Model file for the job. Use its own axes, mm. Face numbers are marked on the shaded views. Round coordinates to 2 decimals unless told otherwise and drop trailing zeros. Write each loop counter-clockwise with the first axis right and the second up, starting at its lowest first coordinate (ties: lowest second). Pieces come first, ordered by that corner, then holes. Notation, with made-up numbers: (52.25, -34.5) - (63.25, -34.5) arc R24 cw to (63.25, -7.5) - close; hole circle Ø3 at (18.25, 73). An arc over 180 degrees is marked (long way). One line per item, written item: value.
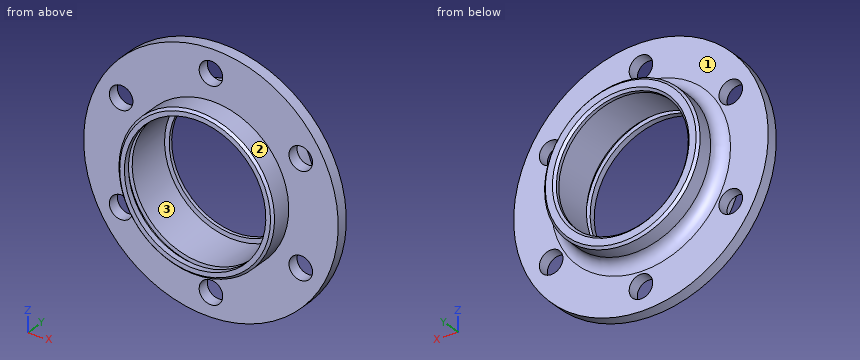
from build123d import *

# Parameters (mm, degrees)
SKETCH1_R           = 27
SKETCH1_R_2         = 2.5
SKETCH1_R_3         = 16.5
BOSS_EXTRUDE1_DEPTH = 2.5
FILLET1_R           = 2.5


with BuildPart() as part:
    # Sketch1 → Boss-Extrude1 (new body)
    with BuildSketch(Plane(origin=(0, 0, 0), x_dir=(1, 0, 0), z_dir=(0, 1, 0))):
        with Locations(Location((0, 0, 0), (0, 0, 270))):
            Circle(SKETCH1_R)
        with Locations(Location((0, 22, 0), (0, 0, 270))):
            Circle(SKETCH1_R_2, mode=Mode.SUBTRACT)
        with Locations(Location((19.052558883, 11, 0), (0, 0, 270))):
            Circle(SKETCH1_R_2, mode=Mode.SUBTRACT)
        with Locations(Location((19.052558883, -11, 0), (0, 0, 270))):
            Circle(SKETCH1_R_2, mode=Mode.SUBTRACT)
        with Locations(Location((0, -22, 0), (0, 0, 270))):
            Circle(SKETCH1_R_2, mode=Mode.SUBTRACT)
        with Locations(Location((-19.052558883, -11, 0), (0, 0, 270))):
            Circle(SKETCH1_R_2, mode=Mode.SUBTRACT)
        with Locations(Location((-19.052558883, 11, 0), (0, 0, 270))):
            Circle(SKETCH1_R_2, mode=Mode.SUBTRACT)
        with Locations(Location((0, 0, 0), (0, 0, 270))):
            Circle(SKETCH1_R_3, mode=Mode.SUBTRACT)
    extrude(amount=-BOSS_EXTRUDE1_DEPTH)

    # Sketch4 → Revolve1 (revolve)
    with BuildSketch(Plane(origin=(0, 0, 0), x_dir=(0, 0, -1), z_dir=(1, 0, 0))):
        Polygon((-16.5, -6.89), (-16.5, 5.75), (-16, 6.25), (-14.992862102, 6.25), (-14.5, 6.25), (-14, 5.75), (-14, 5), (-15, 5), (-15, -5), (-15.855, -5), (-15.855, -6.14), (-15, -6.14), (-15, -7.39), (-16, -7.39), align=None)
    revolve(axis=Axis((0, 12.74988571, 0), (0, -1, 0)))

    # Fillet1
    fillet1_edges = [part.edges().sort_by_distance(p)[0] for p in [
        (0, 0, -16.5),
    ]]
    fillet(fillet1_edges, radius=FILLET1_R)


solid = part.part
1. Mould opens along Z. For the marked faces 1, 2 and 3 say: released by +Z, released by -Z, zero draft, split by the parting line, or undercut.
Report:
face 1: zero draft
face 2: split by the parting line
face 3: undercut
2. Band-saw the part on A-A on z = 22. Write the cut outline in (x, y).
Report:
outline: (-15.65, -2.5) - (-2.5, -2.5) - (-2.5, 0) - (-15.65, 0) - close; (2.5, -2.5) - (15.65, -2.5) - (15.65, 0) - (2.5, 0) - close
3. Band-saw the part on B-B on y = -0.75. Write the cut outline in (x, z).
Report:
outline: circle Ø54 at (0, 0); hole circle Ø5 at (-19.05, -11); hole circle Ø5 at (-19.05, 11); hole circle Ø30 at (0, 0); hole circle Ø5 at (0, -22); hole circle Ø5 at (0, 22); hole circle Ø5 at (19.05, -11); hole circle Ø5 at (19.05, 11)
4. Band-saw the part on D-D on z = 10.5. State how many separate pieces and enclosed holes the cut face has, plus the area to 3 significant figures.
Report:
separate pieces: 4
enclosed holes: 0
area: 94.6 mm²
5. Drop flat-ended pins along their axis: pin 1 (1 mm diameter, centred on x = 15.5, y = -1.5, fed in from +Z); pin 2 (1.5 mm diameter, centred on y = 0.5, z = 15, fed in from -X); pin 3 (8 mm diameter, centred on x = 0, z = 22, fed in from +Y). Give the stop position or say it passes through.
Report:
pin 1: z = 22.45
pin 2: x = -22.81
pin 3: y = 0.21
6. Wall check: probe 1 along X at (y, z) = (-1.55, 11); probe 2 along Z at (x, y) = (0, -5.7) (3 decimals); probe 3 along Z at (x, y) = (0, -6.55). Give the ranges that are in metal, low to high. Write a range as [from, to].
Report:
probe 1: [-24.66, -21.55], [-16.55, -10.2], [10.2, 16.55], [21.55, 24.66]
probe 2: [-16.5, -15.855], [15.855, 16.5]
probe 3: [-16.5, -15], [15, 16.5]
7. Band-saw the part on C-C on y = 4. Write the cut outline in (x, z), plus the area to 3 significant figures.
Report:
outline: circle Ø33 at (0, 0); hole circle Ø30 at (0, 0)
area: 148 mm²
